from build123d import *

# Parameters (mm, degrees)
SKETCH1_R           = 25
BOSS_EXTRUDE1_DEPTH = 10
FILLET1_R           = 5
SKETCH2_R           = 1.5
CUT_EXTRUDE1_DEPTH  = 37.74234621
SKETCH3_R           = 20
CUT_EXTRUDE2_DEPTH  = 5


with BuildPart() as part:
    # Sketch1 → Boss-Extrude1 (new body)
    with BuildSketch(Plane(origin=(0, 0, 0), x_dir=(1, 0, 0), z_dir=(0, 1, 0))):
        with Locations(Location((0, 0, 0), (0, 0, 270))):
            Circle(SKETCH1_R)
    extrude(amount=BOSS_EXTRUDE1_DEPTH)

    # Fillet1
    fillet1_edges = [part.edges().sort_by_distance(p)[0] for p in [
        (0, 10, -25),
    ]]
    fillet(fillet1_edges, radius=FILLET1_R)

    # Sketch2 → Cut-Extrude1 (cut, through all)
    with BuildSketch(Plane(origin=(0, 10, 0), x_dir=(1, 0, 0), z_dir=(0, 1, 0))):
        with Locations(Location((-10, 10, 0), (0, 0, 270))):
            Circle(SKETCH2_R)
        with Locations(Location((10, 10, 0), (0, 0, 270))):
            Circle(SKETCH2_R)
        with Locations(Location((-10, -10, 0), (0, 0, 270))):
            Circle(SKETCH2_R)
        with Locations(Location((10, -10, 0), (0, 0, 270))):
            Circle(SKETCH2_R)
    extrude(amount=-CUT_EXTRUDE1_DEPTH, mode=Mode.SUBTRACT)

    # Sketch3 → Cut-Extrude2 (cut)
    with BuildSketch(Plane.XZ):
        with Locations(Location((0, 0, 0), (0, 0, 270))):
            Circle(SKETCH3_R)
    extrude(amount=-CUT_EXTRUDE2_DEPTH, mode=Mode.SUBTRACT)


solid = part.part
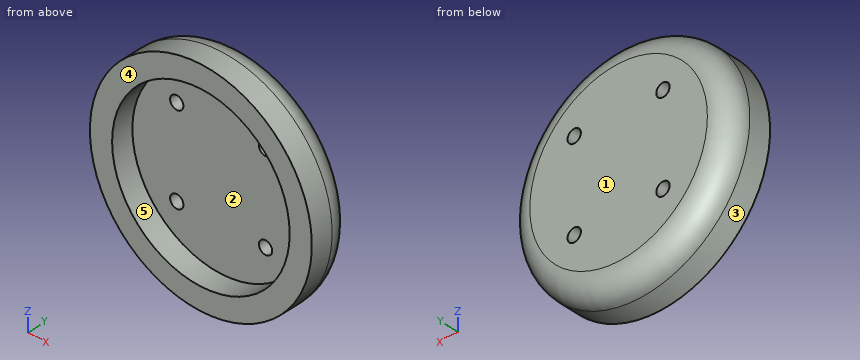
Model file for the job. Use its own axes, mm. Face numbers are marked on the shaded views. A direction names the side the tool comes from. Round coordinates to 2 decimals unless told otherwise and drop trailing zeros. Loops run counter-clockwise (first coordinate to the right, second up) from the corner with the lowest first, then second, coordinate; pieces in that order, holes last. Notation, with made-up numbers: (35, -19.75) -> (53, -19.75) arc R20 cw to (53, 11.25) -> close; hole circle Ø9 at (24, 8.25). An arc over 180 degrees is marked (long way). Answer as CSV lines item,"result". Start each with the question number.
1) Slice it at B-B (y = 9). List the corners of the cut face in (x, z), plus the area to 3 significant figures.
2) Mould opens along Z. For the marked faces 1, 2 and 3 say: +Z half, -Z half, draft (parallel to the pull), parting line (faces both ways), or undercut.
3) Probe line 1 along X through (y, z) = (2.75, 0); line 2 along X through (y, z) = (6.9, 10); line 3 along Y through (x, z) = (-2, -5). List the from-to ranges inside material, lowest first.
4) Tool access for the marked faces 4 and 5: list every direction of +Z, -Z, +X, -X, +Y, -Y with a clear straight run to the whole face (end or side of a thin tool).
5) Slice it at C-C (z = 0). List the corners of the cut face in (x, y).
6) Slice it at D-D (y = 1.75). List the corners of the cut face in (x, z).
7) Pin check, flat tips, straight feed: P1, Ø1.5, axis at y = 5.5, z = 20, coming from the +X side; P2, Ø8, axis at x = 5, z = -10, coming from the -Y side; P3, Ø4, axis at y = 3.5, z = 5.5, coming from the +X side; P4, Ø10, axis at x = -13.5, z = 17.5, coming from the -Y side. Stop position of each tip, or through.
8) Slice it at A-A (x = 0). List the corners of the cut face in (y, z), plus the area to 3 significant figures.
Filled in:
1,outline,"circle Ø46 at (0, 0); hole circle Ø3 at (-10, -10); hole circle Ø3 at (-10, 10); hole circle Ø3 at (10, -10); hole circle Ø3 at (10, 10)"
1,area,"1,630 mm2"
2,face 1,"draft"
2,face 2,"undercut"
2,face 3,"parting line"
3,line 1,"x = -25 to -20, 20 to 25"
3,line 2,"x = -22.5 to -11.5, -8.5 to 8.5, 11.5 to 22.5"
3,line 3,"y = 5 to 10"
4,face 4,"+Z, -Z, +X, -X, -Y"
4,face 5,"-Y"
5,outline,"(-25, 0) -> (-20, 0) -> (-20, 5) -> (20, 5) -> (20, 0) -> (25, 0) -> (25, 5) arc R5 ccw to (20, 10) -> (-20, 10) arc R5 ccw to (-25, 5) -> close"
6,outline,"circle Ø50 at (0, 0); hole circle Ø40 at (0, 0)"
7,P1,"stops at x = 15.92"
7,P2,"stops at y = 5"
7,P3,"stops at x = 24.75"
7,P4,"stops at y = 0"
8,outline,"(0, -25) -> (5, -25) arc R5 ccw to (10, -20) -> (10, 20) arc R5 ccw to (5, 25) -> (0, 25) -> (0, 20) -> (5, 20) -> (5, -20) -> (0, -20) -> close"
8,area,"289 mm2"
